Design review of the part built by this model. Coordinates are the model's own, in mm. Face numbers are marked on the shaded views. Coordinates: 2 decimals unless noted, no trailing zeros. Write each loop counter-clockwise with the first axis right and the second up, starting at its lowest first coordinate (ties: lowest second). Pieces come first, ordered by that corner, then holes.
Q1. The part is to be moulded in two halves that separate along X. For the marked faces 1 and 2, say which applies: released by +X, released by -X, zero draft, split by the parting line, or undercut.
Q2. For pin 1 Ø5 at (y, z) = (53.5, -9.5) entering from -X; pin 2 Ø2 at (y, z) = (7.5, 30) entering from +X; pin 3 Ø8 at (y, z) = (-31.5, 19.5) entering from -X, all flat-tipped, find the tip position at first contact; note any pin that passes through.
Q3. Take a section at A-A, the plane z = 0. Write out the cut boundary in (x, y).
Q4. Take a section at B-B, the plane x = 0. Write out the cut boundary in (y, z), plus the area to 3 significant figures.
Q5. Take a section at C-C, the plane y = 80. Write out the cut boundary in (x, z).
Q6. Take a section at D-D, the plane z = 10. Write out the cut boundary in (x, y).
Q7. For L1, parallel to X at y = 28, z = -1.5; L2, parallel to X at y = 79, z = 0; L3, parallel to Y at x = 0, z = 41, list the stretches that pass through material, from the lowest coordinate up.
from build123d import *

# Parameters (mm, degrees)
SKETCH1_R           = 43.25
SKETCH1_R_2         = 38.25
BOSS_EXTRUDE1_DEPTH = 92.5
BOSS_EXTRUDE2_START = -6.35
SKETCH2_R           = 38.25
SKETCH2_R_2         = 36.25
BOSS_EXTRUDE2_DEPTH = 100
CUT_EXTRUDE3_START  = -44
SKETCH6_R           = 39.25
SKETCH6_R_2         = 38.25
CUT_EXTRUDE3_DEPTH  = 44
SKETCH8_R           = 17.5
CUT_EXTRUDE5_DEPTH  = 111.893530019


with BuildPart() as part:
    # Sketch1 → Boss-Extrude1 (new, symmetric)
    with BuildSketch(Plane(origin=(0, 0, 0), x_dir=(1, 0, 0), z_dir=(0, 1, 0))):
        with Locations(Location((0, 0, 0), (0, 0, 270))):
            Circle(SKETCH1_R)
        with Locations(Location((0, 0, 0), (0, 0, 270))):
            Circle(SKETCH1_R_2, mode=Mode.SUBTRACT)
    extrude(amount=BOSS_EXTRUDE1_DEPTH, both=True)

    # Sketch2 → Boss-Extrude2 (add)
    with BuildSketch(Plane.XZ.offset(92.5).offset(BOSS_EXTRUDE2_START)):
        with Locations(Location((0, 0, 0), (0, 0, 270))):
            Circle(SKETCH2_R)
        with Locations(Location((0, 0, 0), (0, 0, 270))):
            Circle(SKETCH2_R_2, mode=Mode.SUBTRACT)
    extrude(amount=-BOSS_EXTRUDE2_DEPTH)

    # Sketch6 → Cut-Extrude3 (cut)
    with BuildSketch(Plane(origin=(0, 92.5, 0), x_dir=(1, 0, 0), z_dir=(0, 1, 0)).offset(CUT_EXTRUDE3_START)):
        with Locations(Location((0, 0, 0), (0, 0, 270))):
            Circle(SKETCH6_R)
        with Locations(Location((0, 0, 0), (0, 0, 90))):
            Circle(SKETCH6_R_2, mode=Mode.SUBTRACT)
    extrude(amount=CUT_EXTRUDE3_DEPTH, mode=Mode.SUBTRACT)

    # Sketch8 → Cut-Extrude5 (cut, through all)
    with BuildSketch(Plane.XY):
        with Locations(Location((0, 44.35, 0), (0, 0, 90))):
            Circle(SKETCH8_R)
    extrude(amount=CUT_EXTRUDE5_DEPTH, mode=Mode.SUBTRACT)


solid = part.part
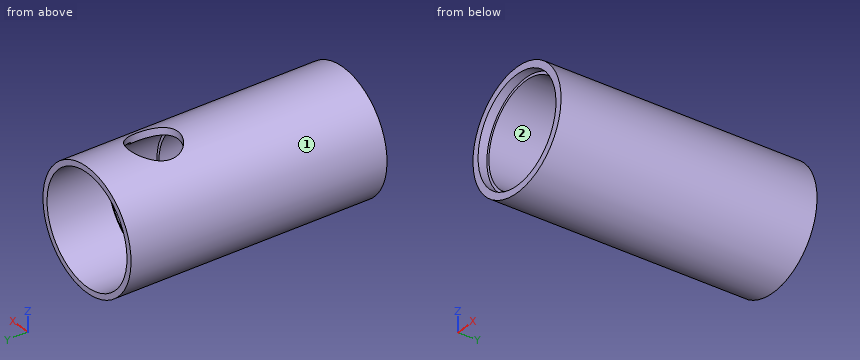
Responses:
1. face 1: split by the parting line
1. face 2: undercut
2. pin 1: stops at x = -42.68
2. pin 2: stops at x = 32.09
2. pin 3: stops at x = -40.38
3. outline: (-43.25, -92.5) - (-38.25, -92.5) - (-38.25, -86.15) - (-36.25, -86.15) - (-36.25, 13.85) - (-38.25, 13.85) - (-38.25, 48.5) - (-39.25, 48.5) - (-39.25, 92.5) - (-43.25, 92.5) - close; (36.25, -86.15) - (38.25, -86.15) - (38.25, -92.5) - (43.25, -92.5) - (43.25, 92.5) - (39.25, 92.5) - (39.25, 48.5) - (38.25, 48.5) - (38.25, 13.85) - (36.25, 13.85) - close
4. outline: (-92.5, -43.25) - (92.5, -43.25) - (92.5, -39.25) - (48.5, -39.25) - (48.5, -38.25) - (13.85, -38.25) - (13.85, -36.25) - (-86.15, -36.25) - (-86.15, -38.25) - (-92.5, -38.25) - close; (-92.5, 38.25) - (-86.15, 38.25) - (-86.15, 36.25) - (13.85, 36.25) - (13.85, 38.25) - (26.85, 38.25) - (26.85, 43.25) - (-92.5, 43.25) - close; (61.85, 39.25) - (92.5, 39.25) - (92.5, 43.25) - (61.85, 43.25) - close
4. area: 2,000 mm2
5. outline: circle Ø86.5 at (0, 0); hole circle Ø78.5 at (0, 0)
6. outline: (-42.08, -92.5) - (-36.92, -92.5) - (-36.92, -86.15) - (-34.84, -86.15) - (-34.84, 13.85) - (-36.92, 13.85) - (-36.92, 48.5) - (-37.95, 48.5) - (-37.95, 92.5) - (-42.08, 92.5) - close; (34.84, -86.15) - (36.92, -86.15) - (36.92, -92.5) - (42.08, -92.5) - (42.08, 92.5) - (37.95, 92.5) - (37.95, 48.5) - (36.92, 48.5) - (36.92, 13.85) - (34.84, 13.85) - close
7. L1: x = -43.22 to -38.22, 38.22 to 43.22
7. L2: x = -43.25 to -39.25, 39.25 to 43.25
7. L3: y = -92.5 to 26.85, 61.85 to 92.5
